Answer from the drawing. Dimensions are ordinates in mm from the lowest x, y and z of the part. A direction names the side the tool comes from. Round coordinates to 2 decimals unless told otherwise and drop trailing zeros. Loops run counter-clockwise (first coordinate to the right, second up) from the corner with the lowest first, then second, coordinate; pieces in that order, holes last. Notation, with made-up numbers: M -13,21.5 L 16,21.5 A13 cw 16,43.5 Z; hole C 46.5,59 d2. An arc over 180 degrees is marked long. One line per item, written item: value.
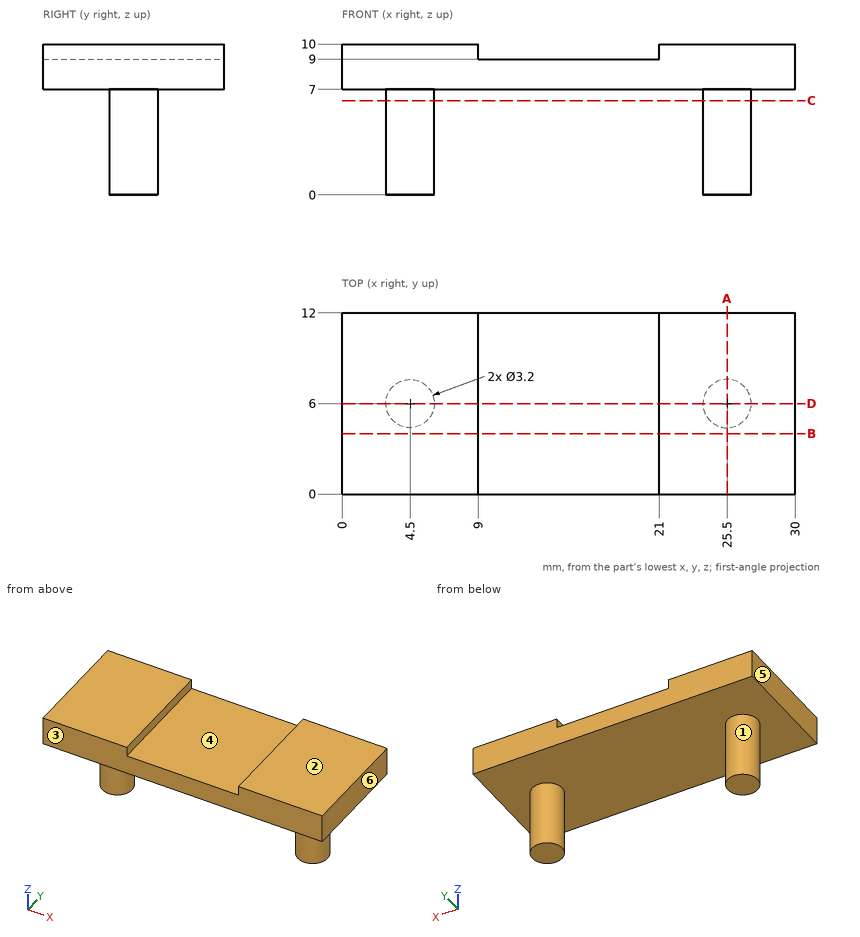
1) Find section C-C (z = 6.25). Give the vertices of the cut face in (x, y), then the cut area to 3 significant figures.
Check values:
outline: C 4.5,6 d3.2; C 25.5,6 d3.2
area: 16.1 mm2
2) Find section A-A (x = 25.5). Give the vertices of the cut face in (y, z).
Check values:
outline: M 0,7 L 4.4,7 L 4.4,0 L 7.6,0 L 7.6,7 L 12,7 L 12,10 L 0,10 Z
3) The mould has two halves that part along X. Classify the marked faces 3, 4, 5 and 6: +X half, -X half, draft (parallel to the pull), parting line (faces both ways), or undercut.
Check values:
face 3: draft
face 4: undercut
face 5: -X half
face 6: +X half
4) Each of these flat-tipped pins is pushed along its axis until it touches: pin 1 (3 mm diameter, centred on y = 7.5, z = 4.5, fed in from +X); pin 2 (4 mm diameter, centred on x = 24, z = 3, fed in from +Y); pin 3 (6 mm diameter, centred on x = 17.5, y = 8, fed in from -Z). Where does it stop, or does it pass through?
Check values:
pin 1: x = 27.1
pin 2: y = 7.6
pin 3: z = 7
5) Find section D-D (y = 6). Give the vertices of the cut face in (x, z), then the cut area to 3 significant figures.
Check values:
outline: M 0,7 L 2.9,7 L 2.9,0 L 6.1,0 L 6.1,7 L 23.9,7 L 23.9,0 L 27.1,0 L 27.1,7 L 30,7 L 30,10 L 21,10 L 21,9 L 9,9 L 9,10 L 0,10 Z
area: 123 mm2
6) Find section B-B (y = 4). Give the vertices of the cut face in (x, z), then the cut area to 3 significant figures.
Check values:
outline: M 0,7 L 30,7 L 30,10 L 21,10 L 21,9 L 9,9 L 9,10 L 0,10 Z
area: 78.0 mm2
7) For the marked faces 1 and 2, determine the directions among +Z, -Z, +X, -X, +Y, -Y from which every point of the face is accessible in a straight line to the end or side of a thin tool.
Check values:
face 1: -Z
face 2: +Z, +X, -X, +Y, -Y
8) Find the intervals of material crossed by probe 1 along Z at (x, y) = (17.75, 6.25); probe 2 along Z at (x, y) = (5.5, 1.5); probe 3 along X at (y, z) = (7, 3.5), in increasing order. Write a range as from..to.
Check values:
probe 1: 7..9
probe 2: 7..10
probe 3: 3.25..5.75, 24.25..26.75
